Job drawing, mm, ordinate dimensions from the low corner. One solid piece. A direction names the side the tool comes from. Round coordinates to 2 decimals unless told otherwise and drop trailing zeros. Write each loop counter-clockwise with the first axis right and the second up, starting at its lowest first coordinate (ties: lowest second). Pieces come first, ordered by that corner, then holes. Notation, with made-up numbers: (-36.5, 27) - (-8.5, 27) arc R26 ccw to (-8.5, 44) - close; hole circle Ø8 at (62, 74). An arc over 180 degrees is marked (long way). Write each question's results on one line, items separated by ' | '.
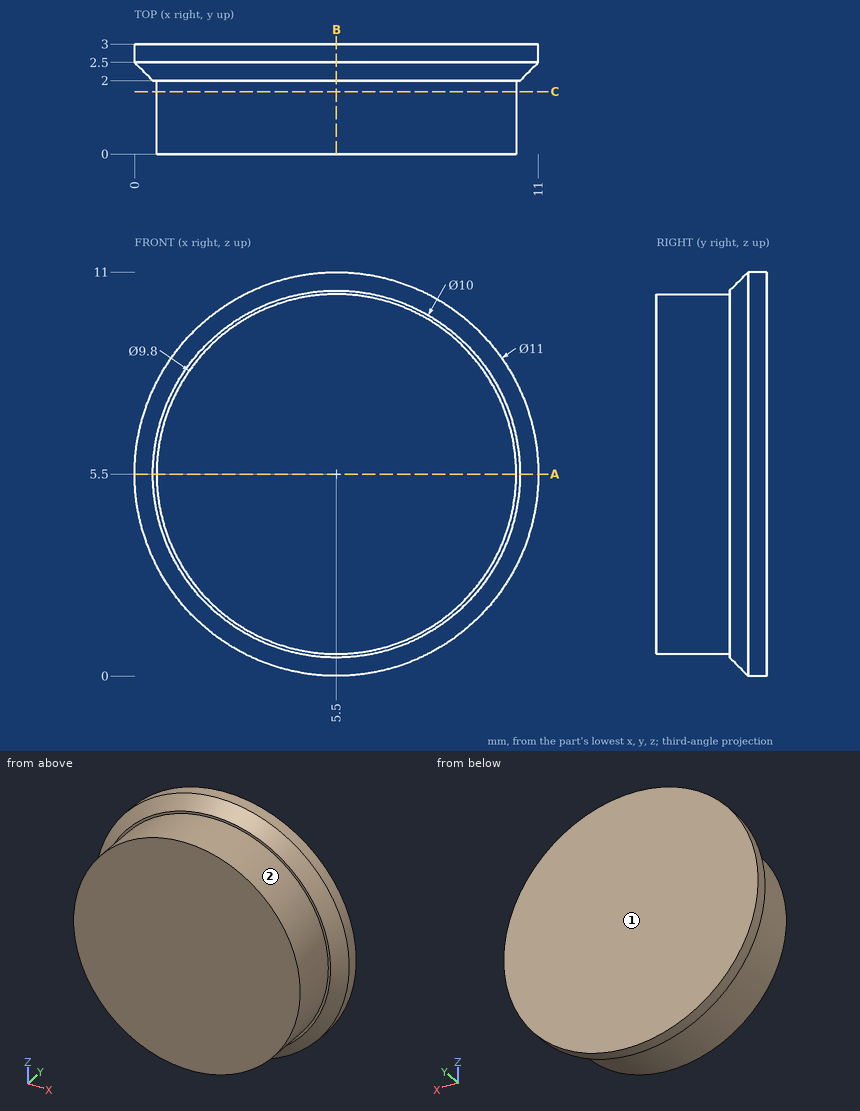
(1) Slice it at A-A, the plane z = 5.5. Write the cut outline in (x, y).
Worked answers:
outline: (0, 2.5) - (0.5, 2) - (0.6, 2) - (0.6, 0) - (10.4, 0) - (10.4, 2) - (10.5, 2) - (11, 2.5) - (11, 3) - (0, 3) - close
(2) Drill centre lines: probe 1 along Y at (x, z) = (10.25, 7); probe 2 along X at (y, z) = (2.6, 4.5); probe 3 along X at (y, z) = (2.25, 9.5). Where is each one in solid material? Low to high. Write a range as [from, to].
Worked answers:
probe 1: y = [2, 3] | probe 2: x = [0.09, 10.91] | probe 3: x = [2.1, 8.9]
(3) Slice it at C-C, the plane y = 1.7. Write the cut outline in (x, z), and give its area (3 significant figures).
Worked answers:
outline: circle Ø9.8 at (5.5, 5.5) | area: 75.4 mm2
(4) Flat gauge pins, fed straight in: pin 1 Ø1.5 at (x, y) = (8.5, 1) entering from +Z; pin 2 Ø1.5 at (x, y) = (2.5, 1) entering from -Z; pin 3 Ø1.5 at (y, z) = (2, 3) entering from -X. Where does each tip first touch, or does it go through?
Worked answers:
pin 1: stops at z = 9.85 | pin 2: stops at z = 1.15 | pin 3: stops at x = 0.35
(5) Tool access for the marked faces 1 and 2: list every direction of +Z, -Z, +X, -X, +Y, -Y with a clear straight run to the whole face (end or side of a thin tool).
Worked answers:
face 1: +Z, -Z, +X, -X, +Y | face 2: -Y
(6) Slice it at B-B, the plane x = 5.5. Write the cut outline in (y, z).
Worked answers:
outline: (0, 0.6) - (2, 0.6) - (2, 0.5) - (2.5, 0) - (3, 0) - (3, 11) - (2.5, 11) - (2, 10.5) - (2, 10.4) - (0, 10.4) - close
